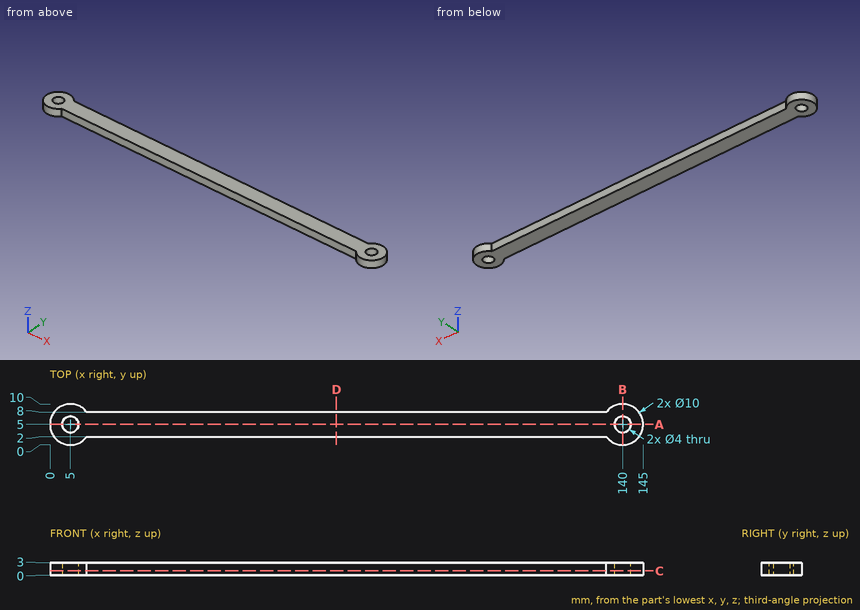
Could you check a few things on this drawing? It's one solid part, dimensions in mm from its lowest x, y, z. Give positions to 0.01 mm unless a question says otherwise; leave off trailing zeros. Order: outer loops, then holes, each group sorted by start corner. A loop starts at its lowest first (then second) coordinate and runs counter-clockwise, first axis right, second up.
1. For pin 1 (0.9 mm diameter, centred on x = 64.5, z = 1.5, fed in from -Y); pin 2 (3.5 mm diameter, centred on x = 140, y = 5, fed in from -Z); pin 3 (1.5 mm diameter, centred on y = 7.5, z = 0.5, fed in from +X), each with a flat end and sliding along its axis, tell me the tip position at first contact or that it passes through.
Answers below:
pin 1: stops at y = 2
pin 2: passes through
pin 3: stops at x = 144.68
2. Suppose I cut it at D-D (x = 70). Write out the boundary of the cut face in (y, z), plus the area to 3 significant figures.
Answers below:
outline: (2, 0) - (8, 0) - (8, 3) - (2, 3) - close
area: 18.0 mm2
3. Suppose I cut it at A-A (y = 5). Write out the boundary of the cut face in (x, z).
Answers below:
outline: (0, 0) - (3, 0) - (3, 3) - (0, 3) - close; (7, 0) - (138, 0) - (138, 3) - (7, 3) - close; (142, 0) - (145, 0) - (145, 3) - (142, 3) - close
4. I need wall thicknesses on L1, parallel to Y at x = 5, z = 1.8; L2, parallel to X at y = 3.5, z = 2.65; L3, parallel to X at y = 4, z = 2.2. Which ranges of each line are inside material? Lowest first, please.
Answers below:
L1: y = 0 to 3, 7 to 10
L2: x = 0.23 to 3.68, 6.32 to 138.68, 141.32 to 144.77
L3: x = 0.1 to 3.27, 6.73 to 138.27, 141.73 to 144.9
5. Suppose I cut it at B-B (x = 140). Write out the boundary of the cut face in (y, z), plus the area to 3 significant figures.
Answers below:
outline: (0, 0) - (3, 0) - (3, 3) - (0, 3) - close; (7, 0) - (10, 0) - (10, 3) - (7, 3) - close
area: 18.0 mm2
6. Suppose I cut it at C-C (z = 1.05). Write out the boundary of the cut face in (x, y).
Answers below:
outline: (9, 2) - (136, 2) arc R5 ccw (long way) to (136, 8) - (9, 8) arc R5 ccw (long way) to start; hole circle Ø4 at (5, 5); hole circle Ø4 at (140, 5)
